Verification items for the finished model (mm, model axes). A direction names the side the tool comes from. Coordinates: 2 decimals unless noted, no trailing zeros. Order: outer loops, then holes, each group sorted by start corner. A loop starts at its lowest first (then second) coordinate and runs counter-clockwise, first axis right, second up.
Q1. Set-up check for faces 1 (the cylindrical face through (-16.85, 19.07, 3.92)), 2 (the flat face through (-15.049, 16.095, 1.38)): record each of +Z, -Z, +X, -X, +Y, -Y from which the full face is reachable in a straight line by a thin tool's end or side.
Q2. Depth check by flat-ended pin: P1, Ø5.5, axis at x = 17.5, y = -17.5, coming from the -Z side; P2, Ø4, axis at x = 23, z = 3.5, coming from the +Y side; P3, Ø6.5, axis at x = -18, y = 16.5, coming from the -Z side; P4, Ø2.5, axis at x = -17.5, y = 17.5, coming from the +Z side. Enter the tip coordinate at first touch or a pass-through.
Q3. Cross-section at A-A, the plane x = 0. Record the boundary of the cut face in (y, z), and give its area (3 significant figures).
Q4. Cross-section at C-C, the plane y = -1. Record the boundary of the cut face in (x, z).
Q5. Draft check along X on faces 3 (the flat face through (19.964, -16.117, 1.38)), 4 (the cylindrical face through (-29.97, -1.32, 2.46)), 5 (the flat face through (0, -6, 5)). Enter one of: pulls with the +X half, pulls with the -X half, needs draft (parallel to the pull), parting line crosses it, or undercut.
Q6. Cross-section at B-B, the plane z = 3.75. Record the boundary of the cut face in (x, y), and give its area (3 significant figures).
Q7. Thickness scan on line 1 (X direction, y = -17.5, z = 3.85); line 2 (Y direction, x = 0, z = 3). Record the ranges inside material, lowest first.
Q8. Cross-section at D-D, the plane x = -17.5. Record the boundary of the cut face in (y, z), and give its area (3 significant figures).
Autodesk Inventor part; units mm, degrees
ref_plane "YZ Plane" through (0, 0, 0) normal (1, 0, 0) x (0, 1, 0)
ref_plane "XZ Plane" through (0, 0, 0) normal (0, 1, 0) x (-1, 0, 0)
ref_plane "XY Plane" through (0, 0, 0) normal (0, 0, 1) x (1, 0, 0)
sketch "Sketch1" plane through (0, 0, 0) normal (0, 0, 1) x (1, 0, 0)
  circle A0 centre (0, 0) radius 30
  dimension "d0" = 60
extrude "Main Body" add sketch "Sketch1" along normal blind 5
sketch "Sketch7" plane through (0, 0, 0) normal (0, 0, -1) x (-1, 0, 0)
  circle A0 centre (0, 0) radius 30
  circle A1 centre (0, 0) radius 10
  dimension "d32" = 20
extrude "Raised Centre" add sketch "Sketch7" along normal blind 3 contours A1
sketch "Sketch8" plane through (0, 0, -3) normal (0, 0, -1) x (-1, 0, 0)
  circle A0 centre (0, 0) radius 10
hole "Centre Hole" at (0, 0, -3) direction (0, 0, 1) diameter 8.4 end through all
sketch "Sketch10" plane through (0, 0, 0) normal (0, 0, -1) x (-1, 0, 0)
  circle A0 centre (0, 0) radius 30
  line L0 (-17.5, 17.5) -> (17.5, 17.5) construction
  line L1 (17.5, 17.5) -> (17.5, -17.5) construction
  line L2 (17.5, -17.5) -> (-17.5, -17.5) construction
  line L3 (-17.5, -17.5) -> (-17.5, 17.5) construction
  line L4 (-17.5, 17.5) -> (17.5, -17.5) construction
  line L5 (17.5, 17.5) -> (-17.5, -17.5) construction
  dimension "d55" = 35
  dimension "d56" = 35
hole "Mount Holes" at (17.5, 17.5, 0) at (-17.5, 17.5, 0) at (-17.5, -17.5, 0) at (17.5, -17.5, 0) direction (0, 0, 1) diameter 3.4 end through all
sketch "Sketch11" plane through (0, 0, 0) normal (0, 0, -1) x (-1, 0, 0)
  circle A0 centre (17.5, -17.5) radius 1.7
  circle A1 centre (-17.5, 17.5) radius 1.7
  circle A2 centre (17.5, 17.5) radius 1.7
  circle A3 centre (-17.5, -17.5) radius 1.7
  line L0 (-15.9008, 14.6569) -> (-19.1627, 14.6935)
  line L1 (-19.1627, 14.6935) -> (-20.7618, 17.5367)
  line L2 (-20.7618, 17.5367) -> (-19.0992, 20.3431)
  line L3 (-19.0992, 20.3431) -> (-15.8373, 20.3065)
  line L4 (-15.8373, 20.3065) -> (-14.2382, 17.4633)
  line L5 (-14.2382, 17.4633) -> (-15.9008, 14.6569)
  line L6 (19.0992, 14.6569) -> (15.8373, 14.6935)
  line L7 (15.8373, 14.6935) -> (14.2382, 17.5367)
  line L8 (14.2382, 17.5367) -> (15.9008, 20.3431)
  line L9 (15.9008, 20.3431) -> (19.1627, 20.3065)
  line L10 (19.1627, 20.3065) -> (20.7618, 17.4633)
  line L11 (20.7618, 17.4633) -> (19.0992, 14.6569)
  line L12 (-15.8575, -20.3184) -> (-19.1195, -20.3316)
  line L13 (-19.1195, -20.3316) -> (-20.762, -17.5132)
  line L14 (-20.762, -17.5132) -> (-19.1425, -14.6816)
  line L15 (-19.1425, -14.6816) -> (-15.8805, -14.6684)
  line L16 (-15.8805, -14.6684) -> (-14.238, -17.4868)
  line L17 (-14.238, -17.4868) -> (-15.8575, -20.3184)
  line L18 (19.1425, -20.3184) -> (15.8805, -20.3316)
  line L19 (15.8805, -20.3316) -> (14.238, -17.5132)
  line L20 (14.238, -17.5132) -> (15.8575, -14.6816)
  line L21 (15.8575, -14.6816) -> (19.1195, -14.6684)
  line L22 (19.1195, -14.6684) -> (20.762, -17.4868)
  line L23 (20.762, -17.4868) -> (19.1425, -20.3184)
  dimension "d64" = 5.65
  dimension "d65" = 5.65
  dimension "d66" = 5.65
  dimension "d67" = 5.65
extrude "Nut Traps" cut sketch "Sketch11" against normal blind 2.8
properties part number "Spool Boss"
Check values:
1. face 1: +Z, -Z
1. face 2: -Z
2. P1: stops at z = 2.8
2. P2: stops at y = 21.42
2. P3: stops at z = 0
2. P4: passes through
3. outline: (-30, 0) - (-10, 0) - (-10, -3) - (-4.2, -3) - (-4.2, 5) - (-30, 5) - close; (4.2, -3) - (10, -3) - (10, 0) - (30, 0) - (30, 5) - (4.2, 5) - close
3. area: 293 mm2
4. outline: (-29.98, 0) - (-9.95, 0) - (-9.95, -3) - (-4.08, -3) - (-4.08, 5) - (-29.98, 5) - close; (4.08, -3) - (9.95, -3) - (9.95, 0) - (29.98, 0) - (29.98, 5) - (4.08, 5) - close
5. face 3: undercut
5. face 4: parting line crosses it
5. face 5: needs draft
6. outline: circle Ø60 at (0, 0); hole circle Ø3.4 at (-17.5, -17.5); hole circle Ø3.4 at (-17.5, 17.5); hole circle Ø8.4 at (0, 0); hole circle Ø3.4 at (17.5, -17.5); hole circle Ø3.4 at (17.5, 17.5)
6. area: 2,740 mm2
7. line 1: x = -24.37 to -19.2, -15.8 to 15.8, 19.2 to 24.37
7. line 2: y = -30 to -4.2, 4.2 to 30
8. outline: (-24.37, 0) - (-20.33, 0) - (-20.33, 2.8) - (-19.2, 2.8) - (-19.2, 5) - (-24.37, 5) - close; (-15.8, 2.8) - (-14.67, 2.8) - (-14.67, 0) - (14.67, 0) - (14.67, 2.8) - (15.8, 2.8) - (15.8, 5) - (-15.8, 5) - close; (19.2, 2.8) - (20.33, 2.8) - (20.33, 0) - (24.37, 0) - (24.37, 5) - (19.2, 5) - close
8. area: 197 mm2
